```python
from build123d import *

# Parameters (mm, degrees)
BOSS_EXTRUDE1_DEPTH = 15
SKETCH2_R           = 3
SKETCH2_W           = 3
SKETCH2_H           = 10
CUT_EXTRUDE1_DEPTH  = 5
FILLET1_R           = 5


with BuildPart() as part:
    # Sketch1 → Boss-Extrude1 (new body)
    with BuildSketch(Plane(origin=(0, 0, 0), x_dir=(1, 0, 0), z_dir=(0, 1, 0))):
        Polygon((-61.880536913, 28.790268456), (-61.880536913, -26.209731544), (-56.880536913, -26.209731544), (-56.880536913, 23.790268456), (-56.880536913, 28.790268456), align=None)
    extrude(amount=BOSS_EXTRUDE1_DEPTH)

    # Sketch2 → Cut-Extrude1 (cut)
    with BuildSketch(Plane.ZY.offset(61.880536913)):
        with Locations((21.209731544, 7.5)):
            Circle(SKETCH2_R)
        with Locations((-25.290268456, 7.5)):
            Rectangle(SKETCH2_W, SKETCH2_H)
    extrude(amount=-CUT_EXTRUDE1_DEPTH, mode=Mode.SUBTRACT)

    # Fillet1
    fillet1_edges = [part.edges().sort_by_distance(p)[0] for p in [
        (-59.380536913, 15, 26.209731544),
        (-59.380536913, 0, 26.209731544),
    ]]
    fillet(fillet1_edges, radius=FILLET1_R)


solid = part.part
```
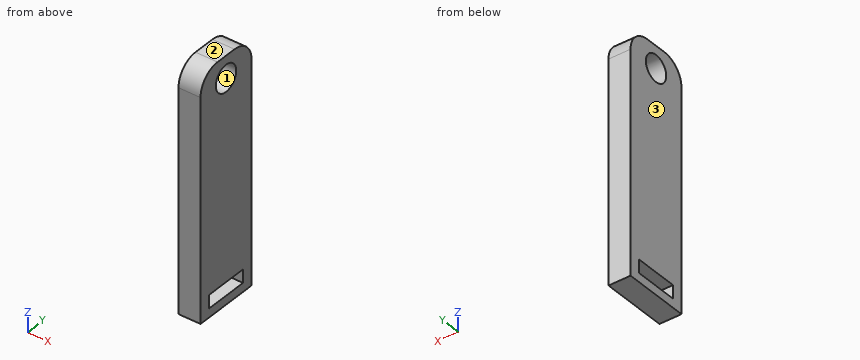
Could you check a few things on this model? Use its own coordinates, in mm. Face numbers are marked on the shaded views. Round coordinates to 2 decimals unless told otherwise and drop trailing zeros. Order: outer loops, then holes, each group sorted by start corner. A loop starts at its lowest first (then second) coordinate and runs counter-clockwise, first axis right, second up. Notation, with made-up numbers: M -5,5.5 L 39,5.5 A16 ccw 39,18.5 Z; hole C -4,-32 d10. An arc over 180 degrees is marked long. One line per question, with ' | ' between items. Start each with the question number.
(1) Suppose I cut it at C-C on y = 13. List the corners of the cut face in (x, z) for me, then the cut area to 3 significant figures.
(2) Suppose I cut it at A-A on x = -57.65. List the corners of the cut face in (y, z) for me.
(3) Thinking about a two-plate mould opening in Z: for the marked faces 1, 2 and 3, which applies, +Z half, -Z half, draft (parallel to the pull), parting line (faces both ways), or undercut?
(4) Please list where these lines run through material, in increasing order: line 1 along Z through (x, y) = (-58.25, 7.75); line 2 along Y through (x, z) = (-60.95, -25.5); line 3 along Z through (x, y) = (-57.55, 5.75).
(5) For P1, Ø3.5, axis at y = 7.5, z = 21.21, coming from the -X side, with a flat end and sliding along its axis, tell me the tip position at first contact or that it passes through.
(6) Suppose I cut it at B-B on y = 7.5. List the corners of the cut face in (x, z) for me.
Geometry results:
1) outline: M -61.88,-28.79 L -56.88,-28.79 L -56.88,25.21 L -61.88,25.21 Z | area: 270 mm²
2) outline: M 0,-28.79 L 15,-28.79 L 15,21.21 A5 ccw 10,26.21 L 5,26.21 A5 ccw 0,21.21 Z; hole M 2.5,-26.79 L 12.5,-26.79 L 12.5,-23.79 L 2.5,-23.79 Z; hole C 7.5,21.21 d6
3) face 1: undercut | face 2: +Z half | face 3: draft
4) line 1: -28.79 to -26.79, -23.79 to 18.22, 24.2 to 26.21 | line 2: 0 to 2.5, 12.5 to 15 | line 3: -28.79 to -26.79, -23.79 to 18.77, 23.65 to 26.21
5) P1: through
6) outline: M -61.88,-28.79 L -56.88,-28.79 L -56.88,-26.79 L -61.88,-26.79 Z; M -61.88,-23.79 L -56.88,-23.79 L -56.88,18.21 L -61.88,18.21 Z; M -61.88,24.21 L -56.88,24.21 L -56.88,26.21 L -61.88,26.21 Z
